The listing builds one solid part. Answer for the finished solid, in the listing's coordinates (mm). Face numbers are marked on the shaded views. A direction names the side the tool comes from. Round coordinates to 2 decimals unless told otherwise and drop trailing zeros. Loops run counter-clockwise (first coordinate to the right, second up) from the corner with the lowest first, then second, coordinate; pieces in that order, holes last. Notation, with made-up numbers: (30.25, -7.5) - (78.25, -7.5) arc R18 ccw to (78.25, -2.5) - close; hole circle Ø1 at (25, 5). An arc over 180 degrees is marked (long way). One line per item, written item: value.
```python
from build123d import *

# Parameters (mm, degrees)
F0_W     = 1.6
F0_H     = 12.5
F0_W_2   = 12.5
F0_H_2   = 1.6
F1_DEPTH = 1
F2_R     = 10
F3_DEPTH = 3.2
F4_COUNT = 4
F5_W     = 3.2
F5_H     = 2
F6_DEPTH = 0.5
F7_COUNT = 4


# Not quite as in the source:
# - a feature names something its author has since deleted; it is built from what else it names


with BuildPart() as f1:
    # F0 (on Top) → F1 (new body)
    with BuildSketch(Plane.XY):
        Polygon((3.1, 14.1), (1.6, 15.6), (1.6, 3.1), (1.6, 1.6), (3.1, 1.6), (15.6, 1.6), (14.1, 3.1), (3.1, 3.1), align=None)
        with Locations((0.8, 9.35)):
            Rectangle(F0_W, F0_H)
        Polygon((1.6, 1.6), (1.6, 3.1), (0, 3.1), (0, 0), (3.1, 0), (3.1, 1.6), align=None)
        with Locations((9.35, 0.8)):
            Rectangle(F0_W_2, F0_H_2)
    extrude(amount=-F1_DEPTH)

    # F2
    f2_edges = [f1.edges().sort_by_distance(p)[0] for p in [
        (3.1, 3.1, -0.5),
    ]]
    fillet(f2_edges, radius=F2_R)

    # F0 (on Top) → F3 (join)
    with BuildSketch(Plane.XY):
        Polygon((3.1, 14.1), (1.6, 15.6), (1.6, 3.1), (1.6, 1.6), (3.1, 1.6), (15.6, 1.6), (14.1, 3.1), (3.1, 3.1), align=None)
        Polygon((1.6, 1.6), (1.6, 3.1), (0, 3.1), (0, 0), (3.1, 0), (3.1, 1.6), align=None)
    extrude(amount=F3_DEPTH)

    # F4: F1 ×4 about axis
    f4_axis = Axis((0, 0, -0.5), (0, 0, 1))


with BuildPart() as f1_1:
    add(f1.part)
    for i in range(1, F4_COUNT):
        add(f1.part.rotate(f4_axis, i * 360 / F4_COUNT))



with BuildPart() as f6:
    # F5 (on face) → F6 (new body)
    with BuildSketch(Plane.XY.offset(3.2)):
        Polygon((1.6, 15.6), (-1.6, 15.6), (-3.1, 14.1), (-3.1, 3.1), (0, 0), (3.1, 3.1), (3.1, 14.1), align=None)
        with Locations((0, 4.1)):
            Rectangle(F5_W, F5_H, mode=Mode.SUBTRACT)
    extrude(amount=F6_DEPTH)


with BuildPart() as f1_2:
    add(f1_1.part)

    add(f6.part)  # F7 merges F6
    # F7: F6 ×4 about axis
    f7_axis = Axis((0, 0, 3.45), (0, 0, -1))
    for i in range(1, F7_COUNT):
        add(f6.part.rotate(f7_axis, i * 360 / F7_COUNT))


solid = f1_2.part
```
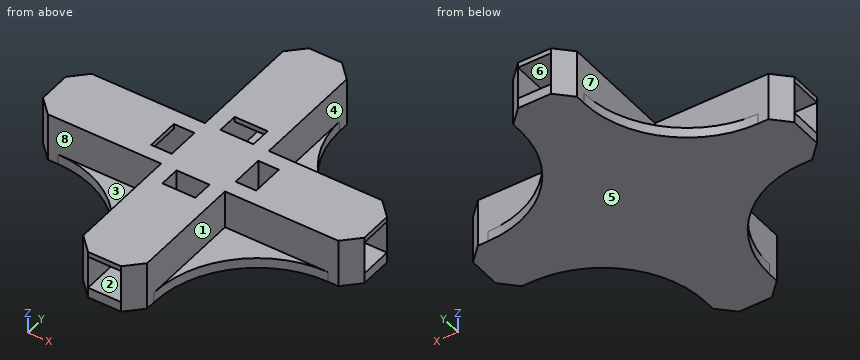
1) For the marked faces 1, 2, 3, 4 and 5, determine the directions among +Z, -Z, +X, -X, +Y, -Y from which every point of the face is accessible in a straight line to the end or side of a thin tool.
Final values:
face 1: +Z, +X, -Y
face 2: -Y
face 3: +Z, -X, -Y
face 4: +Z, +X, +Y
face 5: -Z, +X, -X, +Y, -Y
2) Consider L1, parallel to Y at x = -6, z = 1.95; L2, parallel to Z at x = 1, y = -10.5. Determine where each line is inside the solid, lowest interval first.
Final values:
L1: -3.1 to -1.6, 1.6 to 3.1
L2: -1 to 0, 3.2 to 3.7
3) A cutting plane is placed at C-C on z = -0.55. Give the vertices of the cut face in (x, y).
Final values:
outline: (-15.6, -1.6) - (-14.1, -3.1) - (-13.1, -3.1) arc R10 cw to (-3.1, -13.1) - (-3.1, -14.1) - (-1.6, -15.6) - (1.6, -15.6) - (3.1, -14.1) - (3.1, -13.1) arc R10 cw to (13.1, -3.1) - (14.1, -3.1) - (15.6, -1.6) - (15.6, 1.6) - (14.1, 3.1) - (13.1, 3.1) arc R10 cw to (3.1, 13.1) - (3.1, 14.1) - (1.6, 15.6) - (-1.6, 15.6) - (-3.1, 14.1) - (-3.1, 13.1) arc R10 cw to (-13.1, 3.1) - (-14.1, 3.1) - (-15.6, 1.6) - close
4) Each of these flat-tipped pins is pushed along its axis until it touches: pin 1 Ø2 at (x, y) = (-7, -7) entering from -Z; pin 2 Ø2.5 at (y, z) = (-9, 0.5) entering from +X; pin 3 Ø1.1 at (x, z) = (-8.5, 1) entering from -Y; pin 4 Ø1.4 at (x, z) = (9.5, 0.5) entering from +Y. Where does it stop, or does it pass through?
Final values:
pin 1: through
pin 2: x = 4.59
pin 3: y = -3.1
pin 4: y = 3.97
5) A cutting plane is placed at A-A on y = 13.5. Give the vertices of the cut face in (x, z).
Final values:
outline: (-3.1, -1) - (3.1, -1) - (3.1, 3.7) - (-3.1, 3.7) - close; hole (-1.6, 0) - (1.6, 0) - (1.6, 3.2) - (-1.6, 3.2) - close
6) A cutting plane is placed at D-D on y = -4. Give the vertices of the cut face in (x, z).
Final values:
outline: (-8.95, -1) - (8.95, -1) - (8.95, 0) - (3.1, 0) - (3.1, 3.7) - (1.6, 3.7) - (1.6, 0) - (-1.6, 0) - (-1.6, 3.7) - (-3.1, 3.7) - (-3.1, 0) - (-8.95, 0) - close
7) A cutting plane is placed at B-B on x = 11.5. Give the vertices of the cut face in (y, z).
Final values:
outline: (-3.23, -1) - (3.23, -1) - (3.23, 0) - (3.1, 0) - (3.1, 3.7) - (-3.1, 3.7) - (-3.1, 0) - (-3.23, 0) - close; hole (-1.6, 0) - (1.6, 0) - (1.6, 3.2) - (-1.6, 3.2) - close
8) For a pull along X with two mould halves and no side action, classify the marked faces 6, 7 and 8 as released by +X, released by -X, zero draft, split by the parting line, or undercut.
Final values:
face 6: undercut
face 7: released by -X
face 8: zero draft
